Here's how the part is built. I have some questions about the finished solid (model axes, mm). Give positions to 0.01 mm unless a question says otherwise; leave off trailing zeros. Write each loop counter-clockwise with the first axis right and the second up, starting at its lowest first coordinate (ties: lowest second). Pieces come first, ordered by that corner, then holes. Notation, with made-up numbers: (-19.75, 49.5) -> (36.25, 49.5) arc R31 cw to (36.25, 73.5) -> close; hole circle Ø8 at (79, 14.25). An arc over 180 degrees is marked (long way). Use CSV: the item, a comma, the result in double quotes. Start each with the question number.
(1) I need wall thicknesses on L1, parallel to Y at x = 0, z = 0.9; L2, parallel to X at y = 19, z = 0.4; L3, parallel to Y at x = 22.5, z = 2.85. Which ranges of each line are inside material? Lowest first, please. Write a range as [from, to].
(2) Suppose I cut it at C-C on y = -5. List the corners of the cut face in (x, z) for me.
(3) Suppose I cut it at D-D on x = -10. List the corners of the cut face in (y, z) for me, plus the area to 3 significant figures.
(4) Suppose I cut it at A-A on y = -20. List the corners of the cut face in (x, z) for me.
(5) For pin 1 Ø2.5 at (x, y) = (0, -5) entering from +Z, with a flat end and sliding along its axis, tell me the tip position at first contact or that it passes through.
(6) Suppose I cut it at B-B on z = 3. Give the number of separate pieces and of enclosed holes in the cut face, plus the area to 3 significant figures.
from build123d import *

# Parameters (mm, degrees)
SKETCH_1_W          = 80
SKETCH_1_H          = 100
SKETCH_1_R          = 1.65
EXTRUDE_1_DEPTH     = 4
SKETCH_3_R          = 21
CUT_EXTRUDE_2_DEPTH = 65.156059729
FILLET_1_R          = 2
SKETCH_2_R          = 1.65
CUT_EXTRUDE_1_DEPTH = 65.156059729
FILLET_2_R          = 20
SKETCH_4_R          = 1.65
CUT_EXTRUDE_3_DEPTH = 65.156059729


with BuildPart() as part:
    # 草图1 → 凸台-拉伸1 (new body)
    with BuildSketch(Plane.XY):
        Rectangle(SKETCH_1_W, SKETCH_1_H)
        with Locations((0, 45)):
            Circle(SKETCH_1_R, mode=Mode.SUBTRACT)
        with Locations((21.650635095, 32.5)):
            Circle(SKETCH_1_R, mode=Mode.SUBTRACT)
        with Locations((21.650635095, 7.5)):
            Circle(SKETCH_1_R, mode=Mode.SUBTRACT)
        with Locations((0, -5)):
            Circle(SKETCH_1_R, mode=Mode.SUBTRACT)
        with Locations((-21.650635095, 7.5)):
            Circle(SKETCH_1_R, mode=Mode.SUBTRACT)
        with Locations((-21.650635095, 32.5)):
            Circle(SKETCH_1_R, mode=Mode.SUBTRACT)
    extrude(amount=EXTRUDE_1_DEPTH)

    # 草图3 → 切除-拉伸2 (cut, through all)
    with BuildSketch(Plane.XY.offset(4)):
        with Locations((0, 20)):
            Circle(SKETCH_3_R)
    extrude(amount=-CUT_EXTRUDE_2_DEPTH, mode=Mode.SUBTRACT)

    # 圆角1
    fillet_1_edges = [part.edges().sort_by_distance(p)[0] for p in [
        (40, -50, 2),
        (-40, -50, 2),
    ]]
    fillet(fillet_1_edges, radius=FILLET_1_R)

    # 草图2 → 切除-拉伸1 (cut, through all)
    with BuildSketch(Plane.XY.offset(4)):
        with Locations((-26, -47)):
            Circle(SKETCH_2_R)
        with Locations(Location((-6, -47, 0), (0, 0, 180))):
            Circle(SKETCH_2_R)
        with Locations((6, -47)):
            Circle(SKETCH_2_R)
        with Locations(Location((26, -47, 0), (0, 0, 180))):
            Circle(SKETCH_2_R)
    extrude(amount=-CUT_EXTRUDE_1_DEPTH, mode=Mode.SUBTRACT)

    # 圆角2
    fillet_2_edges = [part.edges().sort_by_distance(p)[0] for p in [
        (-40, 50, 2),
        (40, 50, 2),
    ]]
    fillet(fillet_2_edges, radius=FILLET_2_R)

    # 草图4 → 切除-拉伸3 (cut, through all)
    with BuildSketch(Plane.XY.offset(4)):
        with Locations((-22.5, -20)):
            Circle(SKETCH_4_R)
        with Locations((-22.5, 60)):
            Circle(SKETCH_4_R)
        with Locations(Location((22.5, -20, 0), (0, 0, 180))):
            Circle(SKETCH_4_R)
        with Locations((22.5, 60)):
            Circle(SKETCH_4_R)
    extrude(amount=-CUT_EXTRUDE_3_DEPTH, mode=Mode.SUBTRACT)


solid = part.part
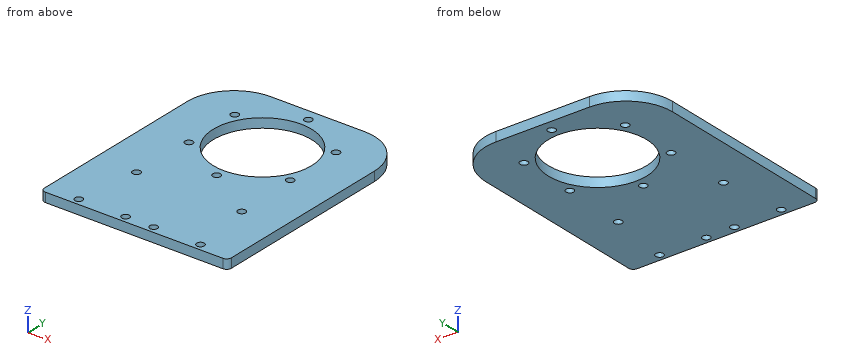
Geometry says:
1,L1,"[-50, -6.65], [-3.35, -1], [41, 43.35], [46.65, 50]"
1,L2,"[-40, -20.98], [20.98, 40]"
1,L3,"[-50, -21.65], [-18.35, 6.09], [8.91, 31.09], [33.91, 49.84]"
2,outline,"(-40, 0) -> (-1.65, 0) -> (-1.65, 4) -> (-40, 4) -> close; (1.65, 0) -> (40, 0) -> (40, 4) -> (1.65, 4) -> close"
3,outline,"(-50, 0) -> (1.53, 0) -> (1.53, 4) -> (-50, 4) -> close; (38.47, 0) -> (50, 0) -> (50, 4) -> (38.47, 4) -> close"
3,area,"252 mm²"
4,outline,"(-40, 0) -> (-24.15, 0) -> (-24.15, 4) -> (-40, 4) -> close; (-20.85, 0) -> (20.85, 0) -> (20.85, 4) -> (-20.85, 4) -> close; (24.15, 0) -> (40, 0) -> (40, 4) -> (24.15, 4) -> close"
5,pin 1,"through"
6,separate pieces,"1"
6,enclosed holes,"13"
6,area,"6,340 mm²"
